Part model, mm, in its own coordinate system. A direction names the side the tool comes from. Round coordinates to 2 decimals unless told otherwise and drop trailing zeros. Loops run counter-clockwise (first coordinate to the right, second up) from the corner with the lowest first, then second, coordinate; pieces in that order, holes last.
(1) Cut at C-C on z = 9.25. List the corners of the cut face in (x, y) (3 decimals).
(2) Probe probe 1 along Z at (x, y) = (-0.25, -6.75); probe 2 along Y at (x, z) = (0, 5.5) (3 decimals); probe 3 along Y at (x, z) = (0, 4.5) (3 decimals). List the from-to ranges inside material, lowest first.
(3) Flat gauge pins, fed straight in: pin 1 (5 mm diameter, centred on y = -5.5, z = 3.5, fed in from -X); pin 2 (1 mm diameter, centred on x = -0.5, y = -1.5, fed in from -Z); pin 3 (2 mm diameter, centred on x = 2.5, z = 2, fed in from -Y). Where does each tip first touch, or does it go through?
(4) Cut at A-A on x = 0. List the corners of the cut face in (y, z) (3 decimals), then the cut area to 3 significant figures.
(5) Tool access for faces 4 (the face through (3.4, 0.1, 12)), 5 (the face through (-0.1, -5.2, 11)): list every direction of +Z, -Z, +X, -X, +Y, -Y with a clear straight run to the whole face (end or side of a thin tool).
(6) Mould opens along Y. For faces 1 (the face through (-0.1, -5.2, 5)), 2 (the face through (-0.69, 3.1, 5.92)), 3 (the face through (-1.09, 4.91, 7.96)) say: +Y half, -Y half, draft (parallel to the pull), parting line (faces both ways), or undercut.
(7) Cut at D-D on x = 3.75. List the corners of the cut face in (y, z), then the cut area to 3 significant figures.
Autodesk Inventor part; units mm, degrees
ref_plane "YZ Plane" through (0, 0, 0) normal (1, 0, 0) x (0, 1, 0)
ref_plane "XZ Plane" through (0, 0, 0) normal (0, 1, 0) x (-1, 0, 0)
ref_plane "XY Plane" through (0, 0, 0) normal (0, 0, 1) x (1, 0, 0)
sketch "Boceto1" plane through (0, 0, 0) normal (0, 0, 1) x (1, 0, 0)
  circle A0 centre (0, 0) radius 8
  circle A1 centre (0, 0) radius 3.175
  dimension "d0" = 16
  dimension "d1" = 6.35
extrude "Extrusión1" add sketch "Boceto1" along normal blind 5
sketch "Boceto2" plane through (0, 0, 5) normal (0, 0, 1) x (1, 0, 0)
  circle A0 centre (0, 0) radius 3.175
  circle A1 centre (0, 0) radius 5.0313
  dimension "d8" = 6.35
extrude "Extrusión2" add sketch "Boceto2" along normal blind 6
sketch "Boceto3" plane through (0, 0, 11) normal (0, 0, 1) x (1, 0, 0)
  circle A0 centre (0, 0) radius 3.175
  circle A1 centre (0, 0) radius 8
  dimension "d9" = 6.35
  dimension "d10" = 16
extrude "Extrusión3" add sketch "Boceto3" along normal blind 1
properties part number "Polea"
Final values:
1. outline: circle Ø10.063 at (0, 0); hole circle Ø6.35 at (0, 0)
2. probe 1: z = 0 to 5, 11 to 12
2. probe 2: y = -5.031 to -3.175, 3.175 to 5.031
2. probe 3: y = -8 to -3.175, 3.175 to 8
3. pin 1: stops at x = -7.42
3. pin 2: passes through
3. pin 3: stops at y = -7.86
4. outline: (-8, 0) - (-3.175, 0) - (-3.175, 12) - (-8, 12) - (-8, 11) - (-5.031, 11) - (-5.031, 5) - (-8, 5) - close; (3.175, 0) - (8, 0) - (8, 5) - (5.031, 5) - (5.031, 11) - (8, 11) - (8, 12) - (3.175, 12) - close
4. area: 80.2 mm2
5. face 4: +Z, +X, -X, +Y, -Y
5. face 5: none
6. face 1: draft
6. face 2: undercut
6. face 3: parting line
7. outline: (-7.07, 0) - (7.07, 0) - (7.07, 5) - (3.35, 5) - (3.35, 11) - (7.07, 11) - (7.07, 12) - (-7.07, 12) - (-7.07, 11) - (-3.35, 11) - (-3.35, 5) - (-7.07, 5) - close
7. area: 125 mm2
